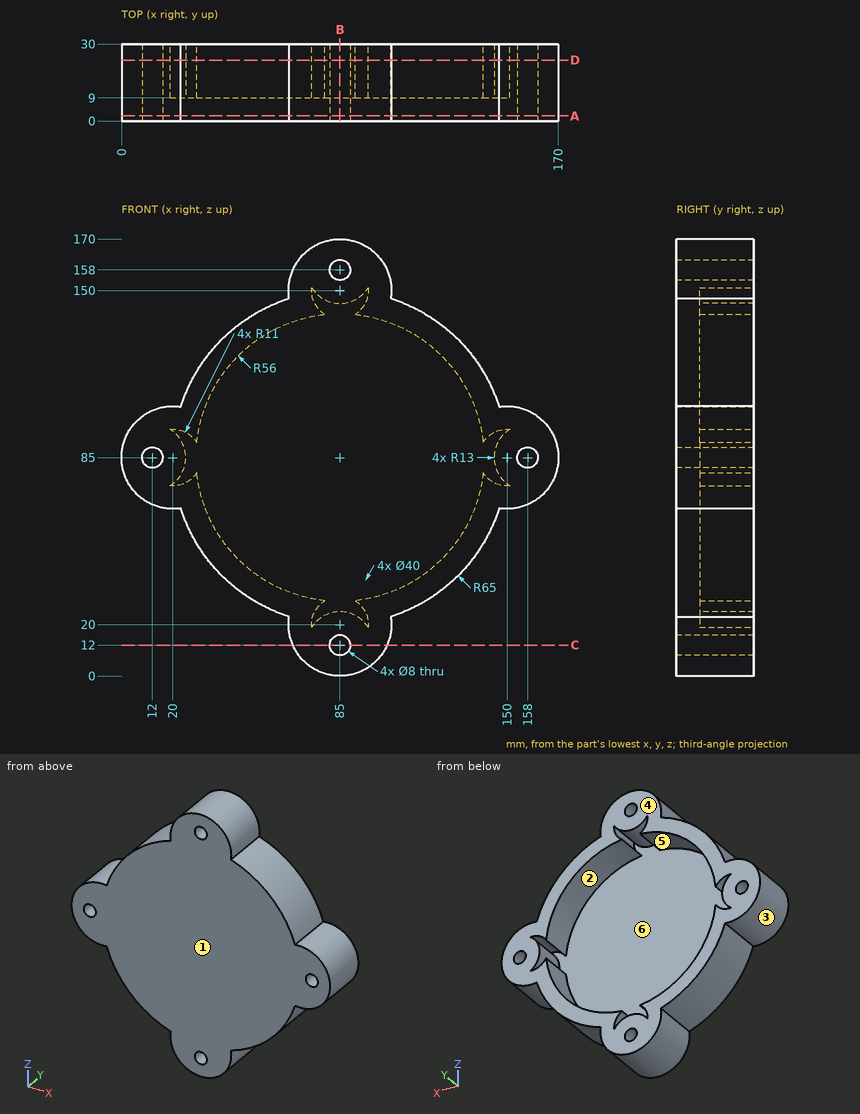
Study the drawing (mm; zero at the part's minimum x, y, z) and answer. A direction names the side the tool comes from. Round coordinates to 2 decimals unless told otherwise and drop trailing zeros. Write each loop counter-clockwise with the first axis right and the second up, starting at its lowest first coordinate (ties: lowest second). Pieces come first, ordered by that corner, then holes. Notation, with made-up numbers: (6.25, 54) -> (56.25, 54) arc R21 cw to (56.25, 75) -> close; hole circle Ø10 at (89.5, -31). An arc over 180 degrees is marked (long way). Use CSV: the item, a comma, the result in double quotes. Start each with the question number.
(1) Which of the six approach directions +Z, -Z, +X, -X, +Y, -Y give full straight-line access (tool end or side, diameter ignored) to the marked faces 1 and 2?
(2) Section D-D on y = 23.75 is taken. Give the vertices of the cut face in (x, z).
(3) Consider L1, parallel to X at y = 13, z = 66.5; L2, parallel to X at y = 14.25, z = 88.5; L3, parallel to Z at x = 58.5, y = 23.5. Determine where each line is inside the solid, lowest interval first. Write a range as from..to.
(4) Section C-C on z = 12 is taken. Give the vertices of the cut face in (x, y), then the cut area to 3 significant figures.
(5) Section B-B on x = 85 is taken. Give the vertices of the cut face in (y, z), then the cut area to 3 significant figures.
(6) Each of these flat-tipped pins is pushed along its axis until it touches: pin 1 (9 mm diameter, centred on x = 12, z = 85, fed in from +Y); pin 2 (3 mm diameter, centred on x = 32.5, y = 20, fed in from +Z); pin 3 (1.5 mm diameter, centred on x = 89, y = 19, fed in from -Z); pin 4 (12 mm diameter, centred on x = 98.5, y = 6, fed in from -Z). Where does it stop, or does it pass through?
(7) The mould has two halves that part along Z. Classify the marked faces 3, 4, 5 and 6: released by +Z, released by -Z, zero draft, split by the parting line, or undercut.
(8) Section A-A on y = 2 is taken. Give the vertices of the cut face in (x, z), then the cut area to 3 significant figures.
A:
1,face 1,"+Z, -Z, +X, -X, -Y"
1,face 2,"+Y"
2,outline,"(23.08, 65.24) arc R65 ccw to (65.24, 23.08) arc R20 ccw (long way) to (104.76, 23.08) arc R65 ccw to (146.92, 65.24) arc R20 ccw (long way) to (146.92, 104.76) arc R65 ccw to (104.76, 146.92) arc R20 ccw (long way) to (65.24, 146.92) arc R65 ccw to (23.08, 104.76) arc R20 ccw (long way) to start; hole circle Ø8 at (12, 85); hole (19, 74.05) arc R11 ccw to (29.31, 79.14) arc R56 ccw to (79.14, 29.31) arc R11 ccw to (74.05, 19) arc R13 cw to (95.95, 19) arc R11 ccw to (90.86, 29.31) arc R56 ccw to (140.69, 79.14) arc R11 ccw to (151, 74.05) arc R13 cw to (151, 95.95) arc R11 ccw to (140.69, 90.86) arc R56 ccw to (90.86, 140.69) arc R11 ccw to (95.95, 151) arc R13 cw to (74.05, 151) arc R11 ccw to (79.14, 140.69) arc R56 ccw to (29.31, 90.86) arc R11 ccw to (19, 95.95) arc R13 cw to start; hole circle Ø8 at (85, 12); hole circle Ø8 at (85, 158); hole circle Ø8 at (158, 85)"
3,L1,"x = 12.4..32.14, 137.86..157.6"
3,L2,"x = 0.31..10.06, 13.94..24.52, 145.48..156.06, 159.94..169.69"
3,L3,"z = 25.65..35.67, 134.33..144.35"
4,outline,"(66.67, 0) -> (81, 0) -> (81, 30) -> (66.67, 30) -> close; (89, 0) -> (103.33, 0) -> (103.33, 30) -> (89, 30) -> close"
4,area,"860 mm²"
5,outline,"(0, 0) -> (30, 0) -> (30, 8) -> (0, 8) -> close; (0, 16) -> (30, 16) -> (30, 25) -> (9, 25) -> (9, 145) -> (30, 145) -> (30, 154) -> (0, 154) -> close; (0, 162) -> (30, 162) -> (30, 170) -> (0, 170) -> close"
5,area,"2,100 mm²"
6,pin 1,"stops at y = 30"
6,pin 2,"stops at z = 125.3"
6,pin 3,"stops at z = 0.27"
6,pin 4,"stops at z = 1.46"
7,face 3,"split by the parting line"
7,face 4,"zero draft"
7,face 5,"undercut"
7,face 6,"undercut"
8,outline,"(23.08, 65.24) arc R65 ccw to (65.24, 23.08) arc R20 ccw (long way) to (104.76, 23.08) arc R65 ccw to (146.92, 65.24) arc R20 ccw (long way) to (146.92, 104.76) arc R65 ccw to (104.76, 146.92) arc R20 ccw (long way) to (65.24, 146.92) arc R65 ccw to (23.08, 104.76) arc R20 ccw (long way) to start; hole circle Ø8 at (12, 85); hole circle Ø8 at (85, 12); hole circle Ø8 at (85, 158); hole circle Ø8 at (158, 85)"
8,area,"15,700 mm²"
